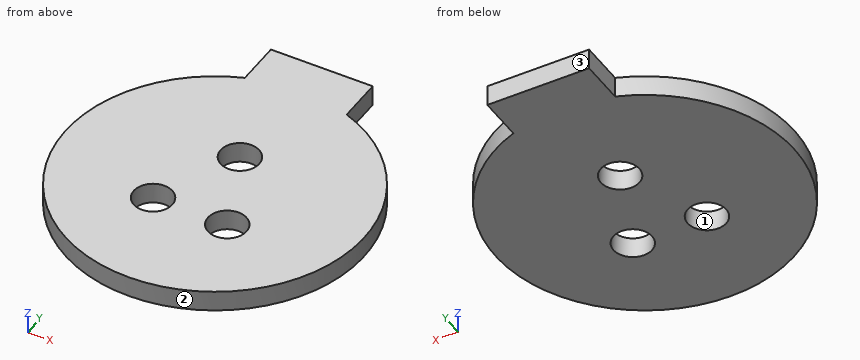
from build123d import *

# Parameters (mm, degrees)
F0_R     = 6.5
F1_DEPTH = 7


with BuildPart() as f1:
    # F0 (on Top) → F1 (new body)
    with BuildSketch(Plane.XY):
        with BuildLine():
            Line((-17.15, 62.456869), (-17.15, 47.216869))
            ThreePointArc((-17.15, 47.216869), (0, -50.235), (17.15, 47.216869))
            Line((17.15, 47.216869), (17.15, 62.456869))
            Line((17.15, 62.456869), (0, 62.456869))
            Line((0, 62.456869), (-17.15, 62.456869))
        make_face()
        with Locations((-12.5, -14.555)):
            Circle(F0_R, mode=Mode.SUBTRACT)
        with Locations((12.5, -14.555)):
            Circle(F0_R, mode=Mode.SUBTRACT)
        with Locations((0, 14.555)):
            Circle(F0_R, mode=Mode.SUBTRACT)
    extrude(amount=F1_DEPTH)


solid = f1.part
Can you work these out from the model? Positions are in its coordinate system, mm. Face numbers are marked on the shaded views. Give positions to 0.01 mm unless a question says otherwise; leave off trailing zeros. Order: outer loops, then holes, each group sorted by start corner. A loop starts at its lowest first (then second) coordinate and runs counter-clockwise, first axis right, second up. Notation, with made-up numbers: M 48,-1.5 L 79,-1.5 A28 ccw 79,19.5 Z; hole C -4.75,-21 d3. An arc over 180 degrees is marked long. One line per question, with ' | ' between items.
Item 1: Suppose I cut it at B-B, the plane z = 3.5. Write out the boundary of the cut face in (x, y) (3 decimals).
Answer block:
outline: M -17.15,47.217 A50.235 ccw long 17.15,47.217 L 17.15,62.457 L -17.15,62.457 Z; hole C -12.5,-14.555 d13; hole C 0,14.555 d13; hole C 12.5,-14.555 d13
Item 2: Suppose I cut it at C-C, the plane y = 49. Write out the boundary of the cut face in (x, z), then the cut area to 3 significant figures.
Answer block:
outline: M -17.15,0 L 17.15,0 L 17.15,7 L -17.15,7 Z | area: 240 mm2
Item 3: We'd pull the mould along X, two halves only. Please class the marked faces 1, 2 and 3: released by +X, released by -X, zero draft, split by the parting line, or undercut.
Answer block:
face 1: undercut | face 2: split by the parting line | face 3: zero draft
Item 4: Please list where these lines run through material, in increasing order: L1, parallel to X at y = -17.5, z = 5.5; L2, parallel to Y at x = 0, z = 2.5 (3 decimals); L3, parallel to X at y = 46.5, z = 1.5.
Answer block:
L1: x = -47.09 to -18.29, -6.71 to 6.71, 18.29 to 47.09 | L2: y = -50.235 to 8.055, 21.055 to 62.457 | L3: x = -19.01 to 19.01
Item 5: Suppose I cut it at D-D, the plane x = 12.5. Write out the boundary of the cut face in (y, z) (3 decimals), then the cut area to 3 significant figures.
Answer block:
outline: M -48.655,0 L -21.055,0 L -21.055,7 L -48.655,7 Z; M -8.055,0 L 62.457,0 L 62.457,7 L -8.055,7 Z | area: 687 mm2
Item 6: Suppose I cut it at A-A, the plane x = 0. Write out the boundary of the cut face in (y, z) (3 decimals).
Answer block:
outline: M -50.235,0 L 8.055,0 L 8.055,7 L -50.235,7 Z; M 21.055,0 L 62.457,0 L 62.457,7 L 21.055,7 Z
Item 7: I'm going to push flat-ended pins straight in: pin 1 Ø2 at (x, z) = (13, 1.5) entering from -Y; pin 2 Ø8 at (x, y) = (0, 14.555) entering from -Z; pin 3 Ø4 at (y, z) = (30.5, 1.5) entering from -X; pin 4 Ø3.5 at (y, z) = (53, 2.5) entering from -X. Where does each tip first touch, or does it pass through?
Answer block:
pin 1: stops at y = -48.78 | pin 2: passes through | pin 3: stops at x = -41.37 | pin 4: stops at x = -17.15
